Check sheet for the drawn part. Datum: minimum x, y, z corner. Units: mm. A direction names the side the tool comes from. Give positions to 0.01 mm unless a question says otherwise; leave off trailing zeros. Loops run counter-clockwise (first coordinate to the right, second up) from the corner with the lowest first, then second, coordinate; pieces in that order, holes last. Notation, with made-up numbers: (-15.5, -36.75) -> (5.5, -36.75) arc R23 ccw to (5.5, 0.25) -> close; hole circle Ø11 at (-33.75, 32.5). An arc over 180 degrees is marked (long way). One line per question, with ' | ' between items.
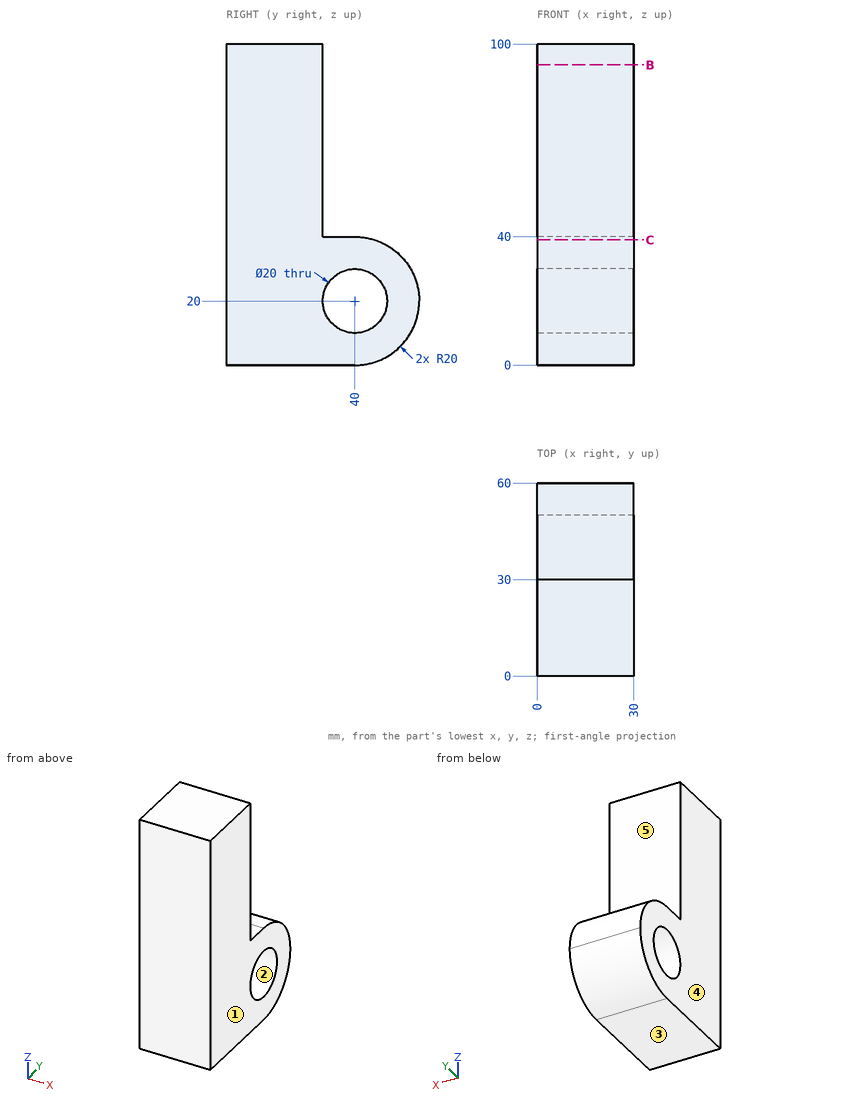
Item 1: Release check for a two-part mould opening along Z. For the marked faces 1, 2 and 3 record: pulls with the +Z half, pulls with the -Z half, needs draft (parallel to the pull), parting line crosses it, or undercut.
Result:
face 1: needs draft | face 2: undercut | face 3: pulls with the -Z half
Item 2: Set-up check for the marked faces 4 and 5: record each of +Z, -Z, +X, -X, +Y, -Y from which the full face is reachable in a straight line by a thin tool's end or side.
Result:
face 4: +Z, -Z, -X, +Y, -Y | face 5: +Z, +X, -X, +Y
Item 3: Sectioned sample at B-B (z = 93.5). Record the cut outline in (x, y), plus the area to 3 significant figures.
Result:
outline: (0, 0) -> (30, 0) -> (30, 30) -> (0, 30) -> close | area: 900 mm2
Item 4: Depth check by flat-ended pin: pin 1 Ø8 at (x, y) = (14.5, 36.5) entering from +Z; pin 2 Ø9 at (x, z) = (21.5, 84) entering from +Y; pin 3 Ø18 at (y, z) = (40, 20) entering from +X. Enter the tip coordinate at first touch or a pass-through.
Result:
pin 1: z = 40 | pin 2: y = 30 | pin 3: through
Item 5: Sectioned sample at C-C (z = 39). Record the cut outline in (x, y) (3 decimals).
Result:
outline: (0, 0) -> (30, 0) -> (30, 46.245) -> (0, 46.245) -> close
Item 6: Scan lines: probe 1 along Z at (x, y) = (22.75, 40); probe 2 along Y at (x, z) = (25.25, 64.5); probe 3 along Z at (x, y) = (6, 35). Record each from-to range of solid material in increasing order.
Result:
probe 1: 0 to 10, 30 to 40 | probe 2: 0 to 30 | probe 3: 0 to 11.34, 28.66 to 40
